Part model, mm, in its own coordinate system. A direction names the side the tool comes from. Give positions to 0.01 mm unless a question says otherwise; leave off trailing zeros. Order: outer loops, then holes, each group sorted by start corner. A loop starts at its lowest first (then second) coordinate and runs counter-clockwise, first axis right, second up. Notation, with made-up numbers: M 44.25,43 L 82.25,43 A20 cw 82.25,54 Z; hole C -5,50 d7. An arc over 180 degrees is marked long. Answer as a JSON object with one key per item and string values.
from build123d import *

# Parameters (mm, degrees)
F0_R     = 2.25
F0_R_2   = 11.2
F1_DEPTH = 6
F2_SIZE  = 0.5
F3_R     = 1


with BuildPart() as f1:
    # F0 (on Top) → F1 (new body)
    with BuildSketch(Plane.XY):
        with BuildLine():
            Line((-17.2, 17.5), (-27.5, 17.5))
            ThreePointArc((-27.5, 17.5), (-31.0355339059, 16.0355339059), (-32.5, 12.5))
            Line((-32.5, 12.5), (-32.5, -9.75))
            Line((-32.5, -9.75), (-28, -9.75))
            ThreePointArc((-28, -9.75), (-26.4090097423, -10.4090097423), (-25.75, -12))
            ThreePointArc((-25.75, -12), (-26.4090097423, -13.5909902577), (-28, -14.25))
            Line((-28, -14.25), (-32.5, -14.25))
            Line((-32.5, -14.25), (-32.5, -17.5))
            Line((-32.5, -17.5), (-17.2, -17.5))
            Line((-17.2, -17.5), (-17.2, -15.5))
            ThreePointArc((-17.2, -15.5), (-15.5, -13.8), (-13.8, -15.5))
            Line((-13.8, -15.5), (-13.8, -17.5))
            Line((-13.8, -17.5), (13.8, -17.5))
            Line((13.8, -17.5), (13.8, -15.5))
            ThreePointArc((13.8, -15.5), (15.5, -13.8), (17.2, -15.5))
            Line((17.2, -15.5), (17.2, -17.5))
            Line((17.2, -17.5), (27.5, -17.5))
            ThreePointArc((27.5, -17.5), (31.0355339059, -16.0355339059), (32.5, -12.5))
            Line((32.5, -12.5), (32.5, 9.75))
            Line((32.5, 9.75), (28, 9.75))
            ThreePointArc((28, 9.75), (25.75, 12), (28, 14.25))
            Line((28, 14.25), (32.5, 14.25))
            Line((32.5, 14.25), (32.5, 17.5))
            Line((32.5, 17.5), (17.2, 17.5))
            Line((17.2, 17.5), (17.2, 15.5))
            ThreePointArc((17.2, 15.5), (15.5, 13.8), (13.8, 15.5))
            Line((13.8, 15.5), (13.8, 17.5))
            Line((13.8, 17.5), (-13.8, 17.5))
            Line((-13.8, 17.5), (-13.8, 15.5))
            ThreePointArc((-13.8, 15.5), (-15.5, 13.8), (-17.2, 15.5))
            Line((-17.2, 15.5), (-17.2, 17.5))
        make_face()
        with Locations((28, -12)):
            Circle(F0_R, mode=Mode.SUBTRACT)
        with Locations((-28, 12)):
            Circle(F0_R, mode=Mode.SUBTRACT)
        Circle(F0_R_2, mode=Mode.SUBTRACT)
    extrude(amount=F1_DEPTH)

    # F2
    f2_edges = [f1.edges().sort_by_distance(p)[0] for p in [
        (-11.2, 0, 6),
        (-11.2, 0, 0),
        (-25.75, -12, 0),
        (-15.5, -13.8, 0),
        (15.5, -13.8, 0),
        (25.75, -12, 0),
        (25.75, 12, 0),
        (15.5, 13.8, 0),
        (-15.5, 13.8, 0),
        (-30.25, 12, 0),
        (-30.25, 12, 6),
        (-15.5, 13.8, 6),
        (15.5, 13.8, 6),
        (25.75, 12, 6),
        (-25.75, -12, 6),
        (-15.5, -13.8, 6),
        (15.5, -13.8, 6),
        (25.75, -12, 6),
        (-13.8, 16.5, 6),
        (-17.2, 16.5, 6),
        (-30.25, -9.75, 6),
        (-30.25, -14.25, 6),
        (-17.2, -16.5, 6),
        (-13.8, -16.5, 6),
        (13.8, -16.5, 6),
        (17.2, -16.5, 6),
        (30.25, 9.75, 6),
        (30.25, 14.25, 6),
        (17.2, 16.5, 6),
        (13.8, 16.5, 6),
        (17.2, 16.5, 0),
        (30.25, 14.25, 0),
        (30.25, 9.75, 0),
        (17.2, -16.5, 0),
        (13.8, -16.5, 0),
        (-13.8, -16.5, 0),
        (-17.2, -16.5, 0),
        (-30.25, -14.25, 0),
        (-30.25, -9.75, 0),
        (-17.2, 16.5, 0),
        (-13.8, 16.5, 0),
        (13.8, 16.5, 0),
    ]]
    chamfer(f2_edges, length=F2_SIZE)

    # F3
    f3_edges = [f1.edges().sort_by_distance(p)[0] for p in [
        (-32.5, -14.25, 3),
        (-32.5, -9.75, 3),
        (-32.5, -17.5, 3),
        (-17.2, -17.5, 3),
        (-13.8, -17.5, 3),
        (13.8, -17.5, 3),
        (17.2, -17.5, 3),
        (32.5, 14.25, 3),
        (32.5, 9.75, 3),
        (32.5, 17.5, 3),
        (17.2, 17.5, 3),
        (13.8, 17.5, 3),
        (-13.8, 17.5, 3),
        (-17.2, 17.5, 3),
    ]]
    fillet(f3_edges, radius=F3_R)


solid = f1.part
1. Cut at A-A on y = 0. Give the cut face in (x, z).
Worked answers:
{"outline": "M -32.5,0 L -11.7,0 L -11.2,0.5 L -11.2,5.5 L -11.7,6 L -32.5,6 Z; M 11.2,0.5 L 11.7,0 L 32.5,0 L 32.5,6 L 11.7,6 L 11.2,5.5 Z"}
2. Pin check, flat tips, straight feed: P1, Ø4, axis at x = 28, y = -12, coming from the +Z side; P2, Ø1.5, axis at y = 12, z = 3.5, coming from the +X side; P3, Ø1.5, axis at y = 13.5, z = 3.5, coming from the -X side; P4, Ø0.8, axis at y = -16, z = 2, coming from the +X side. Stop position of each tip, or through.
Worked answers:
{"P1": "passes through", "P2": "stops at x = 25.88", "P3": "stops at x = -32.49", "P4": "stops at x = 31.42"}
3. Probe line 1 along Y through (x, z) = (0, 2.2); line 2 along Y through (x, z) = (-7, 4.5); line 3 along X through (y, z) = (15, 1.75). List the from-to ranges inside material, lowest first.
Worked answers:
{"line 1": "y = -17.5 to -11.2, 11.2 to 17.5", "line 2": "y = -17.5 to -8.74, 8.74 to 17.5", "line 3": "x = -31.83 to -17.12, -13.88 to 13.88, 17.12 to 32.47"}
4. Cut at B-B on x = 0. Give the cut face in (y, z).
Worked answers:
{"outline": "M -17.5,0 L -11.7,0 L -11.2,0.5 L -11.2,5.5 L -11.7,6 L -17.5,6 Z; M 11.2,0.5 L 11.7,0 L 17.5,0 L 17.5,6 L 11.7,6 L 11.2,5.5 Z"}
5. Two-plate mould, pull along Y, no slides. Class faces 1 (the cylindrical face through (-15.5, 13.8, 3)), 2 (the flat face through (30, 14.25, 3)), 3 (the conical face through (25.61, 11.95, 0.36)), 4 (the conical face through (15.46, -13.66, 0.36)): +Y half, -Y half, draft (parallel to the pull), parting line (faces both ways), or undercut.
Worked answers:
{"face 1": "+Y half", "face 2": "undercut", "face 3": "undercut", "face 4": "-Y half"}
6. Cut at C-C on z = 3. State how many separate pieces and enclosed holes the cut face has, plus the area to 3 significant figures.
Worked answers:
{"separate pieces": "1", "enclosed holes": "3", "area": "1,730 mm^2"}
7. Which spindle directions (+Z, -Z, +X, -X, +Y, -Y) get a long thin tool onto all of the face, cutting with end or side? Do faces 5 (the flat face through (-30, -9.75, 3)), 6 (the cylindrical face through (-15.5, -13.8, 3)). Say none if no direction does.
Worked answers:
{"face 5": "+Z, -Z, -X", "face 6": "+Z, -Z, -Y"}
